The figure shows three views and two pictorial views of one solid part (mm, origin at its lowest corner). Answer the questions. Coordinates: 2 decimals unless noted, no trailing zeros. Loops run counter-clockwise (first coordinate to the right, second up) from the corner with the lowest first, then second, coordinate; pieces in that order, holes last. Notation, with made-up numbers: (-13, 7) -> (31, 7) arc R28 ccw to (31, 35) -> close; hole circle Ø5 at (-25.75, 49.5). An arc over 180 degrees is marked (long way). Use a Markdown table: item, result. Add a question column.
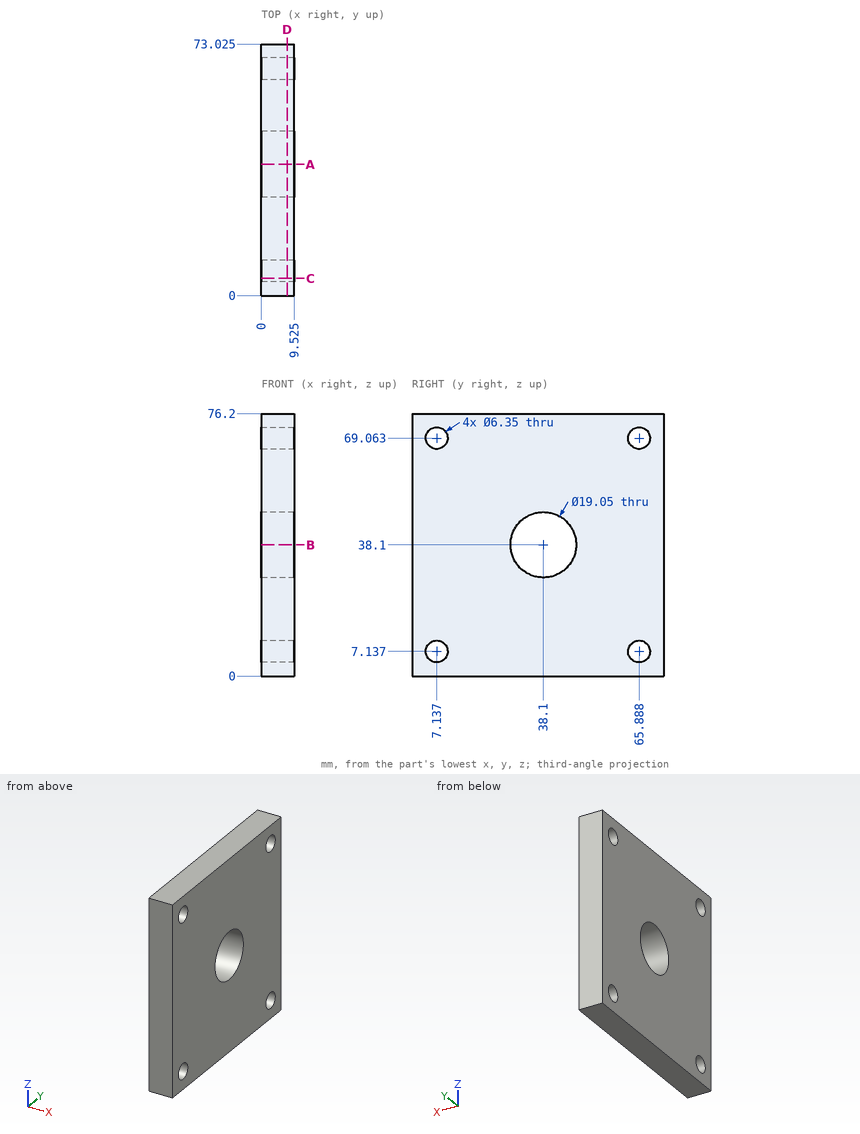
Item 1: Section C-C (y = 5) is taken. Determine the outline of the cut face in (x, z) (1 decimal).
Item 2: Section A-A (y = 38.1) is taken. Determine the outline of the cut face in (x, z) (1 decimal).
Item 3: Given pin 1 (4 mm diameter, centred on y = 65.89, z = 69.06, fed in from -X), flat-ended and moving along its own axis, determine where the tip first touches the part or whether it passes through.
Item 4: Find the intervals of material crossed by probe 1 along Y at (x, z) = (3.75, 38.5) (1 decimal); probe 2 along Z at (x, y) = (5, 9) (1 decimal); probe 3 along Z at (x, y) = (5.5, 6.5), in increasing order.
Item 5: Section B-B (z = 38.1) is taken. Determine the outline of the cut face in (x, y) (1 decimal), then the cut area to 3 significant figures.
Item 6: Section D-D (x = 7.5) is taken. Count the separate pieces of the cut face and the enclosed holes in it, then the cut area to 3 significant figures.
Output:
| question | item | result |
|---|---|---|
| 1 | outline | (0, 0) -> (9.5, 0) -> (9.5, 4.8) -> (0, 4.8) -> close; (0, 9.5) -> (9.5, 9.5) -> (9.5, 66.7) -> (0, 66.7) -> close; (0, 71.4) -> (9.5, 71.4) -> (9.5, 76.2) -> (0, 76.2) -> close |
| 2 | outline | (0, 0) -> (9.5, 0) -> (9.5, 28.6) -> (0, 28.6) -> close; (0, 47.6) -> (9.5, 47.6) -> (9.5, 76.2) -> (0, 76.2) -> close |
| 3 | pin 1 | passes through |
| 4 | probe 1 | y = 0 to 28.6, 47.6 to 73 |
| 4 | probe 2 | z = 0 to 4.6, 9.7 to 66.5, 71.6 to 76.2 |
| 4 | probe 3 | z = 0 to 4.03, 10.25 to 65.95, 72.17 to 76.2 |
| 5 | outline | (0, 0) -> (9.5, 0) -> (9.5, 28.6) -> (0, 28.6) -> close; (0, 47.6) -> (9.5, 47.6) -> (9.5, 73) -> (0, 73) -> close |
| 5 | area | 514 mm2 |
| 6 | separate pieces | 1 |
| 6 | enclosed holes | 5 |
| 6 | area | 5,150 mm2 |
